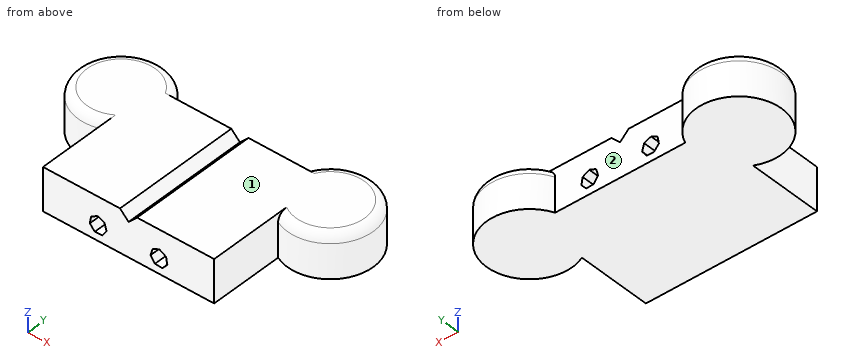
```python
from build123d import *

# Parameters (mm, degrees)
F1_DEPTH = 25.4
F3_DEPTH = 76.2
F4_SIZE  = 5.08
F5_R     = 5.08


with BuildPart() as f1:
    # F0 (on Top) → F1 (new body)
    with BuildSketch(Plane.XY):
        with BuildLine():
            Line((-29.263646, -2.026047), (-29.263646, -45.816111))
            Line((-29.263646, -45.816111), (21.536354, -45.816111))
            Line((21.536354, -45.816111), (21.536354, 30.383889))
            Line((21.536354, 30.383889), (-17.080803, 30.383889))
            ThreePointArc((-17.080803, 30.383889), (-64.345783, 29.655996), (-29.263646, -2.026047))
        make_face()
    extrude(amount=F1_DEPTH)

    # F2 (on face) → F3 (cut)
    with BuildSketch(Plane(origin=(0, 30.383889, 0), x_dir=(-1, 0, 0), z_dir=(0, 1, 0))):
        Polygon((-1.464986, 4.272543), (1.464986, 7.590214), (0.697935, 11.949494), (-3.188536, 14.067755), (-7.267835, 12.349904), (-8.468165, 8.089517), (-5.885655, 4.494753), align=None)
    extrude(amount=-F3_DEPTH, mode=Mode.SUBTRACT)

    # F4
    f4_edges = [f1.edges().sort_by_distance(p)[0] for p in [
        (21.536354, -7.716111, 25.4),
    ]]
    chamfer(f4_edges, length=F4_SIZE)

    # F5
    f5_edges = [f1.edges().sort_by_distance(p)[0] for p in [
        (-64.345783, 29.655996, 25.4),
    ]]
    fillet(f5_edges, radius=F5_R)

    # F6: F1 across face


with BuildPart() as f1_1:
    add(f1.part)
    add(f1.part.mirror(Plane(origin=(21.536354, -7.716111, 10.16), x_dir=(0, 1, 0), z_dir=(1, 0, 0))))


solid = f1_1.part
```
Can you work these out from the model? Positions are in its coordinate system, mm. Face numbers are marked on the shaded views. Coordinates: 2 decimals unless noted, no trailing zeros. Loops run counter-clockwise (first coordinate to the right, second up) from the corner with the lowest first, then second, coordinate; pieces in that order, holes last.
Item 1: Suppose I cut it at B-B (z = 23.5). Please give me the cut outline in (x, y), then the cut area to 3 significant figures.
Answers below:
outline: (-29.26, -45.82) - (18.36, -45.82) - (18.36, 30.38) - (-18.29, 30.38) arc R24.28 ccw (long way) to (-29.26, -0.77) - close; (24.72, -45.82) - (72.34, -45.82) - (72.34, -0.77) arc R24.28 ccw (long way) to (61.37, 30.38) - (24.72, 30.38) - close
area: 10,300 mm2
Item 2: Please list where these lines run through material, in increasing order: L1, parallel to X at y = -8, z = 13; L2, parallel to X at y = 13.5, z = 8.25; L3, parallel to X at y = -27, z = 14.75.
Answers below:
L1: x = -29.26 to 1.23, 5.72 to 37.35, 41.84 to 72.34
L2: x = -64.92 to -1.35, 8.42 to 34.65, 44.42 to 108
L3: x = -29.26 to 72.34
Item 3: Suppose I cut it at A-A (y = -16.5). Please give me the cut outline in (x, z), then the cut area to 3 significant figures.
Answers below:
outline: (-29.26, 0) - (72.34, 0) - (72.34, 25.4) - (26.62, 25.4) - (21.54, 20.32) - (16.46, 25.4) - (-29.26, 25.4) - close; hole (-1.46, 7.59) - (1.46, 4.27) - (5.89, 4.49) - (8.47, 8.09) - (7.27, 12.35) - (3.19, 14.07) - (-0.7, 11.95) - close; hole (34.6, 8.09) - (37.19, 4.49) - (41.61, 4.27) - (44.54, 7.59) - (43.77, 11.95) - (39.88, 14.07) - (35.8, 12.35) - close
area: 2,410 mm2
Item 4: Suppose I cut it at C-C (x = 50). Please give me the cut outline in (y, z), then the cut area to 3 significant figures.
Answers below:
outline: (-45.82, 0) - (30.38, 0) - (30.38, 25.4) - (-45.82, 25.4) - close
area: 1,940 mm2
Item 5: If we mould it in two halves opening along X, with no side actions, what happens to the marked faces 1 and 2? For each: released by +X, released by -X, zero draft, split by the parting line, or undercut.
Answers below:
face 1: zero draft
face 2: undercut
Item 6: Suppose I cut it at D-D (y = 21.5). State how many separate pieces and enclosed holes the cut face has, then the cut area to 3 significant figures.
Answers below:
separate pieces: 1
enclosed holes: 2
area: 4,270 mm2
Item 7: I'm going to push flat-ended pins straight in: pin 1 (12.5 mm diameter, centred on y = -31.5, z = 16.5, fed in from -X); pin 2 (12.5 mm diameter, centred on y = -27.5, z = 7.5, fed in from +X); pin 3 (4 mm diameter, centred on x = 86.5, z = 7.5, fed in from -Y). Where does each tip first touch, or does it pass through?
Answers below:
pin 1: stops at x = -29.26
pin 2: stops at x = 72.34
pin 3: stops at y = -4.67
